Geometry check sheet. Reference: the model listing, model coordinates, mm. Coordinates: 2 decimals unless noted, no trailing zeros. Write each loop counter-clockwise with the first axis right and the second up, starting at its lowest first coordinate (ties: lowest second). Pieces come first, ordered by that corner, then holes. Notation, with made-up numbers: (-2, -9.5) -> (32, -9.5) arc R9 cw to (32, -3.5) -> close; hole circle Ø6 at (77.5, 26.5). An arc over 180 degrees is marked (long way). One line per question, with ' | ' between items.
from build123d import *

# Parameters (mm, degrees)
F1_DEPTH = 3
F3_D     = 3.7
F5_R     = 40
F6_DEPTH = 25
F7_R     = 2
F8_D     = 3.5


with BuildPart() as f1:
    # F0 (on Top) → F1 (new body)
    with BuildSketch(Plane.XY):
        with BuildLine():
            Line((-26.741671, -33.577967), (54.258329, -33.577967))
            ThreePointArc((54.258329, -33.577967), (57.793863, -32.113501), (59.258329, -28.577967))
            Line((59.258329, -28.577967), (59.258329, 92.922033))
            ThreePointArc((59.258329, 92.922033), (57.793863, 96.457566), (54.258329, 97.922033))
            Line((54.258329, 97.922033), (-26.741671, 97.922033))
            ThreePointArc((-26.741671, 97.922033), (-30.277205, 96.457566), (-31.741671, 92.922033))
            Line((-31.741671, 92.922033), (-31.741671, -28.577967))
            ThreePointArc((-31.741671, -28.577967), (-30.277205, -32.113501), (-26.741671, -33.577967))
        make_face()
    extrude(amount=F1_DEPTH)

    # F3 (through all)
    with Locations(Plane.XY.offset(3)):
        with Locations((-24.941671, 91.222033), (52.458329, 91.222033), (52.458329, -26.877967), (-24.941671, -26.877967)):
            Hole(F3_D / 2)

    # F5 (on face) → F6 (cut)
    with BuildSketch(Plane.XY.offset(3)):
        with Locations((13.758329, 32.172033)):
            Circle(F5_R)
    extrude(amount=-F6_DEPTH, mode=Mode.SUBTRACT)

    # F7
    f7_edges = [f1.edges().sort_by_distance(p)[0] for p in [
        (-31.741671, 32.172033, 3),
        (13.758329, 97.922033, 3),
    ]]
    fillet(f7_edges, radius=F7_R)

    # F8 (through all)
    with Locations(Plane.XY.offset(3)):
        with Locations((-22.241671, 68.172033), (49.758329, 68.172033), (49.758329, -3.827967), (-22.241671, -3.827967)):
            Hole(F8_D / 2)


solid = f1.part
1. Cross-section at C-C on x = 10. Record the boundary of the cut face in (y, z), and give its area (3 significant figures).
Worked answers:
outline: (-33.58, 0) -> (-7.65, 0) -> (-7.65, 3) -> (-31.58, 3) arc R2 ccw to (-33.58, 1) -> close; (72, 0) -> (97.92, 0) -> (97.92, 1) arc R2 ccw to (95.92, 3) -> (72, 3) -> close | area: 154 mm²
2. Cross-section at B-B on z = 2.25. Give the number of separate pieces and of enclosed holes in the cut face, and give its area (3 significant figures).
Worked answers:
separate pieces: 1 | enclosed holes: 9 | area: 6,650 mm²
3. Material ranges on line 1 (X direction, y = -3.5, z = 1.8); line 2 (X direction, y = 92, z = 1.6); line 3 (X direction, y = 90.5, z = 0.8), recorded low to high. Write a range as from..to.
Worked answers:
line 1: -31.57..-23.96, -20.52..-4.34, 31.86..48.04, 51.48..59.09 | line 2: -31.65..-26.62, -23.26..50.78, 54.14..59.17 | line 3: -31.74..-26.64, -23.24..50.76, 54.16..59.26
4. Go/stop test with a flat-tipped pin: P1, Ø1.5, axis at x = 32, z = 2.5, coming from the +Y side. Record where the tip stops, or that it passes through.
Worked answers:
P1: y = 97.78
5. Cross-section at A-A on y = 27. Record the boundary of the cut face in (x, z), and give its area (3 significant figures).
Worked answers:
outline: (-31.74, 0) -> (-25.91, 0) -> (-25.91, 3) -> (-29.74, 3) arc R2 ccw to (-31.74, 1) -> close; (53.42, 0) -> (59.26, 0) -> (59.26, 1) arc R2 ccw to (57.26, 3) -> (53.42, 3) -> close | area: 33.3 mm²
6. Mould release check, pull along Y, two halves, no side actions. Record for faces 1 (the face through (32.216, -3.315, 1.521)), 2 (the face through (-30.238, 96.496, 0.493)), 3 (the face through (-16, 5, 3)), 4 (the face through (53.93, 90.1, 1.48)): released by +Y, released by -Y, zero draft, split by the parting line, or undercut.
Worked answers:
face 1: undercut | face 2: released by +Y | face 3: zero draft | face 4: undercut
